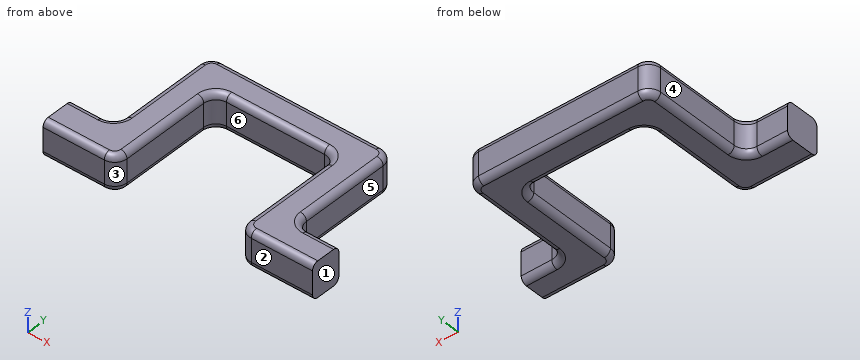
from build123d import *

# Parameters (mm, degrees)
SKETCH3_W           = 29
SKETCH3_H           = 28
BOSS_EXTRUDE2_DEPTH = 60
SKETCH4_W           = 25
SKETCH4_H           = 29
BOSS_EXTRUDE3_DEPTH = 90
SKETCH5_W           = 29
SKETCH5_H           = 25
BOSS_EXTRUDE4_DEPTH = 125
SKETCH7_W           = 25
SKETCH7_H           = 29
BOSS_EXTRUDE5_DEPTH = 93
SKETCH8_W           = 29
SKETCH8_H           = 25
BOSS_EXTRUDE6_DEPTH = 35
FILLET1_R           = 10
FILLET2_R           = 10
FILLET3_R           = 5


with BuildPart() as part:
    # Sketch3 → Boss-Extrude2 (new body)
    with BuildSketch(Plane(origin=(0, 0, 0), x_dir=(0, 0, -1), z_dir=(1, 0, 0))):
        Rectangle(SKETCH3_W, SKETCH3_H)
    extrude(amount=BOSS_EXTRUDE2_DEPTH)

    # Sketch4 → Boss-Extrude3 (add)
    with BuildSketch(Plane(origin=(0, 14, 0), x_dir=(1, 0, 0), z_dir=(0, 1, 0))):
        with Locations((47.5, 0)):
            Rectangle(SKETCH4_W, SKETCH4_H)
    extrude(amount=BOSS_EXTRUDE3_DEPTH)

    # Sketch5 → Boss-Extrude4 (add)
    with BuildSketch(Plane(origin=(60, 0, 0), x_dir=(0, 0, -1), z_dir=(1, 0, 0))):
        with Locations((0, 91.5)):
            Rectangle(SKETCH5_W, SKETCH5_H)
    extrude(amount=BOSS_EXTRUDE4_DEPTH)

    # Sketch7 → Boss-Extrude5 (add)
    with BuildSketch(Plane.XZ.offset(-79)):
        with Locations((172.5, 0)):
            Rectangle(SKETCH7_W, SKETCH7_H)
    extrude(amount=BOSS_EXTRUDE5_DEPTH)

    # Sketch8 → Boss-Extrude6 (add)
    with BuildSketch(Plane(origin=(185, 0, 0), x_dir=(0, 0, -1), z_dir=(1, 0, 0))):
        with Locations((0, -1.5)):
            Rectangle(SKETCH8_W, SKETCH8_H)
    extrude(amount=BOSS_EXTRUDE6_DEPTH)

    # Fillet1
    fillet1_edges = [part.edges().sort_by_distance(p)[0] for p in [
        (35, 14, 0),
        (35, 104, 0),
        (185, 104, 0),
        (160, 79, 0),
        (185, 11, 0),
    ]]
    fillet(fillet1_edges, radius=FILLET1_R)

    # Fillet2
    fillet2_edges = [part.edges().sort_by_distance(p)[0] for p in [
        (60, 79, 0),
        (160, -14, 0),
        (60, -14, 0),
    ]]
    fillet(fillet2_edges, radius=FILLET2_R)

    # Fillet3
    fillet3_edges = [part.edges().sort_by_distance(p)[0] for p in [
        (60, 32.5, 14.5),
        (60, 32.5, -14.5),
        (195, -14, -14.5),
        (160, 32.5, -14.5),
        (25, -14, -14.5),
        (162.928932188, -11.071067812, -14.5),
        (57.071067812, -11.071067812, -14.5),
        (25, -14, 14.5),
        (160, 32.5, 14.5),
        (162.928932188, -11.071067812, 14.5),
        (57.071067812, -11.071067812, 14.5),
        (62.928932188, 76.071067812, -14.5),
        (62.928932188, 76.071067812, 14.5),
        (195, -14, 14.5),
        (207.5, 11, -14.5),
        (207.5, 11, 14.5),
        (110, 79, 14.5),
        (110, 79, -14.5),
        (35, 59, 14.5),
        (35, 59, -14.5),
        (12.5, 14, -14.5),
        (12.5, 14, 14.5),
        (110, 104, 14.5),
        (110, 104, -14.5),
        (185, 57.5, 14.5),
        (182.071067812, 101.071067812, 14.5),
        (37.928932188, 101.071067812, 14.5),
        (185, 57.5, -14.5),
        (182.071067812, 101.071067812, -14.5),
        (37.928932188, 101.071067812, -14.5),
        (157.071067812, 76.071067812, -14.5),
        (157.071067812, 76.071067812, 14.5),
        (32.071067812, 16.928932188, 14.5),
        (32.071067812, 16.928932188, -14.5),
        (187.928932188, 13.928932188, 14.5),
        (187.928932188, 13.928932188, -14.5),
    ]]
    fillet(fillet3_edges, radius=FILLET3_R)


solid = part.part
Model file for the job. Use its own axes, mm. Face numbers are marked on the shaded views. A direction names the side the tool comes from. Give positions to 0.01 mm unless a question says otherwise; leave off trailing zeros. Write each loop counter-clockwise with the first axis right and the second up, starting at its lowest first coordinate (ties: lowest second). Pieces come first, ordered by that corner, then holes. Notation, with made-up numbers: M -2,-5 L 39,-5 A5 cw 39,1 Z; hole C 78,-15 d6. An arc over 180 degrees is marked long. One line per item, written item: value. Start each with the question number.
Q1. Saw through at B-B, the plane x = 93.5. Write the cut outline in (y, z), plus the area to 3 significant figures.
Q2. Drop flat-ended pins along their axis: pin 1 Ø1 at (x, z) = (100.5, 5) entering from -Y; pin 2 Ø12 at (y, z) = (50, 11) entering from +X; pin 3 Ø15 at (y, z) = (29, -4.5) entering from -X; pin 4 Ø10 at (x, z) = (185, 11.5) entering from -Y. Give the stop position or say it passes through.
Q3. Saw through at D-D, the plane y = -1. Write the cut outline in (x, z), plus the area to 3 significant figures.
Q4. Two-plate mould, pull along X, no slides. Class the marked faces 1, 2 and 3: +X half, -X half, draft (parallel to the pull), parting line (faces both ways), or undercut.
Q5. Saw through at C-C, the plane z = -6.75. Write the cut outline in (x, y), plus the area to 3 significant figures.
Q6. 3-axis set-ups, long thin cutter, end or side, ignore diameter. For the marked faces 4, 5 and 6: which of +Z, -Z, +X, -X, +Y, -Y reach the whole face in a straight line?
Q7. Probe probe 1 along X at (y, z) = (40, -8); probe 2 along X at (y, z) = (-2.5, -8); probe 3 along Y at (x, z) = (113.5, -1.5). List the from-to ranges inside material, lowest first. Write a range as [from, to].
Q8. Saw through at A-A, the plane y = 66. Write the cut outline in (x, z), plus the area to 3 significant figures.
Output values:
1. outline: M 79,-9.5 A5 ccw 84,-14.5 L 99,-14.5 A5 ccw 104,-9.5 L 104,9.5 A5 ccw 99,14.5 L 84,14.5 A5 ccw 79,9.5 Z
1. area: 704 mm²
2. pin 1: stops at y = 79
2. pin 2: stops at x = 185
2. pin 3: stops at x = 34.68
2. pin 4: stops at y = -14
3. outline: M 0,-14.5 L 55,-14.5 A5 ccw 60,-9.5 L 60,9.5 A5 ccw 55,14.5 L 0,14.5 Z; M 160,-9.5 A5 ccw 165,-14.5 L 220,-14.5 L 220,14.5 L 165,14.5 A5 ccw 160,9.5 Z
3. area: 3,460 mm²
4. face 1: +X half
4. face 2: draft
4. face 3: undercut
5. outline: M 0,-14 L 50,-14 A10 ccw 60,-4 L 60,69 A10 cw 70,79 L 150,79 A10 cw 160,69 L 160,-4 A10 ccw 170,-14 L 220,-14 L 220,11 L 195,11 A10 cw 185,21 L 185,94 A10 ccw 175,104 L 45,104 A10 ccw 35,94 L 35,24 A10 cw 25,14 L 0,14 Z
5. area: 10,300 mm²
6. face 4: +Z, -Z, -X, +Y
6. face 5: +Z, -Z, +X, +Y
6. face 6: +Z, -Z, -Y
7. probe 1: x = [35, 60], [160, 185]
7. probe 2: x = [0, 60], [160, 220]
7. probe 3: y = [79, 104]
8. outline: M 35,-9.5 A5 ccw 40,-14.5 L 55,-14.5 A5 ccw 60,-9.5 L 60,9.5 A5 ccw 55,14.5 L 40,14.5 A5 ccw 35,9.5 Z; M 160,-9.5 A5 ccw 165,-14.5 L 180,-14.5 A5 ccw 185,-9.5 L 185,9.5 A5 ccw 180,14.5 L 165,14.5 A5 ccw 160,9.5 Z
8. area: 1,410 mm²
